```python
from build123d import *

# Parameters (mm, degrees)
F0_R     = 32.5
F0_R_2   = 18
F1_DEPTH = 39.5


with BuildPart() as f1:
    # F0 (on Front) → F1 (new body)
    with BuildSketch(Plane.XZ):
        Circle(F0_R)
        Circle(F0_R_2, mode=Mode.SUBTRACT)
    extrude(amount=F1_DEPTH)

    # F2 (on Top) → F3 (revolve, cut)
    with BuildSketch(Plane.XY):
        with BuildLine():
            Line((31.389073, -15.398732), (25.373673, -15.398732))
            Line((25.373673, -15.398732), (25.373673, -19.75))
            Line((25.373673, -19.75), (38.296562, -19.75))
            Line((38.296562, -19.75), (38.296562, 9.950572))
            Line((38.296562, 9.950572), (25.373673, 9.950572))
            Line((25.373673, 9.950572), (25.373673, -2.857341))
            ThreePointArc((25.373673, -2.857341), (26.975102, -9.14418), (31.389073, -13.898732))
            Line((31.389073, -13.898732), (31.389073, -15.398732))
        make_face()
    revolve(axis=Axis((5.5, -19.75, 0), (1, 0, 0)), mode=Mode.SUBTRACT)


solid = f1.part
```
Geometry: final body of the model. Coordinates: model frame, mm. A direction names the side the tool comes from. Coordinates: 2 decimals unless noted, no trailing zeros. Order: outer loops, then holes, each group sorted by start corner. A loop starts at its lowest first (then second) coordinate and runs counter-clockwise, first axis right, second up. Notation, with made-up numbers: (55.5, 12.25) - (70.5, 12.25) arc R29 cw to (70.5, 50.25) - close; hole circle Ø4 at (-33, -12). An arc over 180 degrees is marked (long way). Write each question's results on one line, items separated by ' | '.
(1) Section query B-B, the plane x = 0. Return the cut outline in (y, z), plus the area to 3 significant figures.
Values found:
outline: (-39.5, -32.5) - (0, -32.5) - (0, -18) - (-39.5, -18) - close; (-39.5, 18) - (0, 18) - (0, 32.5) - (-39.5, 32.5) - close | area: 1,150 mm²
(2) Section query A-A, the plane z = 0. Return the cut outline in (x, y).
Values found:
outline: (-32.5, -39.5) - (-18, -39.5) - (-18, 0) - (-32.5, 0) - close; (18, -39.5) - (25.37, -39.5) - (25.37, -36.64) arc R13.14 cw to (31.39, -25.6) - (31.39, -24.1) - (25.37, -24.1) - (25.37, -15.4) - (31.39, -15.4) - (31.39, -13.9) arc R13.14 cw to (25.37, -2.86) - (25.37, 0) - (18, 0) - close
(3) Set-up query: faces 4 (the face through (31.389, -24, -2)), 5 (the face through (25.374, -20, 0)). Return all of +Z, -Z, +X, -X, +Y, -Y with unobstructed straight access to the full face (end or side cutting, diameter ignored); none if empty.
Values found:
face 4: +Z, -Z, +X, +Y, -Y | face 5: +X
(4) Section query D-D, the plane x = 17. Return the cut outline in (y, z), plus the area to 3 significant figures.
Values found:
outline: (-39.5, -27.7) - (0, -27.7) - (0, -5.92) - (-39.5, -5.92) - close; (-39.5, 5.92) - (0, 5.92) - (0, 27.7) - (-39.5, 27.7) - close | area: 1,720 mm²
(5) First-contact query: pin 1 Ø4 at (y, z) = (-10, 18.5) entering from -X; pin 2 Ø21.5 at (x, z) = (0, 0) entering from +Y; pin 3 Ø1 at (x, y) = (-6.5, -5) entering from -Z; pin 4 Ø2 at (y, z) = (-12.5, 13) entering from +X. Flat tips, straight axial feed; report the tip coordinate or a pass-through.
Values found:
pin 1: stops at x = -28 | pin 2: passes through | pin 3: stops at z = -31.94 | pin 4: stops at x = 25.72
(6) Mould query, pull axis Y, two halves, no side actions, for faces 1 (the face through (-17, 0, -7)), 2 (the face through (25.374, -2, 0)), 3 (the face through (28.34, -22.96, 2.94)). Classes: +Y half, -Y half, draft (parallel to the pull), parting line (faces both ways), or undercut.
Values found:
face 1: +Y half | face 2: draft | face 3: undercut
(7) Line query: line 1 (X direction, y = -9.5, z = -13.5); line 2 (X direction, y = -7.5, z = 4); line 3 (Z direction, x = -7, y = -7). Output: solid intervals per line, ascending. Write a range as [from, to].
Values found:
line 1: x = [-29.56, -11.91], [11.91, 25.37] | line 2: x = [-32.25, -17.55], [17.55, 26] | line 3: z = [-31.74, -16.58], [16.58, 31.74]
(8) Section query C-C, the plane y = -19.75. Return the cut outline in (x, z), plus the area to 3 significant figures.
Values found:
outline: (25.37, -20.31) - (25.37, -16.89) arc R13.14 cw to (31.39, -5.85) - (31.39, -4.35) - (25.37, -4.35) - (25.37, 4.35) - (31.39, 4.35) - (31.39, 5.85) arc R13.14 cw to (25.37, 16.89) - (25.37, 20.31) arc R32.5 ccw (long way) to start; hole circle Ø36 at (0, 0) | area: 2,160 mm²
